Could you check a few things on this model? Use its own coordinates, in mm. A direction names the side the tool comes from. Coordinates: 2 decimals unless noted, no trailing zeros. Order: outer loops, then holes, each group sorted by start corner. A loop starts at its lowest first (then second) coordinate and runs counter-clockwise, first axis right, second up. Notation, with made-up numbers: M 53,-1.75 L 70,-1.75 A27 cw 70,34.25 Z; hole C -15.75,-18 d6. An arc over 180 degrees is marked long. Put each result on its own line as item: value. Start each with the question number.
```python
from build123d import *

# Parameters (mm, degrees)
SKETCH1_R           = 21.5
SKETCH1_R_2         = 1.55
BOSS_EXTRUDE1_DEPTH = 6
SKETCH2_R           = 5.5
SKETCH2_W           = 20
SKETCH2_H           = 10
CUT_EXTRUDE1_DEPTH  = 12
BOSS_EXTRUDE2_DEPTH = 3
SKETCH4_W           = 2
SKETCH4_H           = 4
BOSS_EXTRUDE3_DEPTH = 3
CHAMFER1_SIZE       = 1
CHAMFER2_SIZE       = 3


with BuildPart() as part:
    # Sketch1 → Boss-Extrude1 (new body)
    with BuildSketch(Plane(origin=(0, 0, 0), x_dir=(1, 0, 0), z_dir=(0, 1, 0))):
        with Locations(Location((0, 0, 0), (0, 0, 270))):
            Circle(SKETCH1_R)
        with Locations(Location((0, 17.320762114, 0), (0, 0, 270))):
            Circle(SKETCH1_R_2, mode=Mode.SUBTRACT)
        with Locations(Location((15, -8.66, 0), (0, 0, 270))):
            Circle(SKETCH1_R_2, mode=Mode.SUBTRACT)
        with Locations(Location((-15, -8.66, 0), (0, 0, 270))):
            Circle(SKETCH1_R_2, mode=Mode.SUBTRACT)
    extrude(amount=BOSS_EXTRUDE1_DEPTH)

    # Sketch2 → Cut-Extrude1 (cut)
    with BuildSketch(Plane(origin=(0, 0, 0), x_dir=(-1, 0, 0), z_dir=(0, -1, 0))):
        with Locations(Location((0, 0, 0), (0, 0, 90))):
            Circle(SKETCH2_R)
        with Locations((0, -17)):
            Rectangle(SKETCH2_W, SKETCH2_H)
    extrude(amount=-CUT_EXTRUDE1_DEPTH, mode=Mode.SUBTRACT)

    # Sketch3 → Boss-Extrude2 (add)
    with BuildSketch(Plane(origin=(0, 6, 0), x_dir=(1, 0, 0), z_dir=(0, 1, 0))):
        with BuildLine():
            ThreePointArc((-5.4375, 0.826797285), (-7, 0), (-5.4375, -0.826797285))
            ThreePointArc((-5.4375, -0.826797285), (-5.5, 0), (-5.4375, 0.826797285))
        make_face()
        with BuildLine():
            ThreePointArc((5.4375, -0.826797285), (7, 0), (5.4375, 0.826797285))
            ThreePointArc((5.4375, 0.826797285), (5.5, 0), (5.4375, -0.826797285))
        make_face()
    extrude(amount=BOSS_EXTRUDE2_DEPTH)

    # Sketch4 → Boss-Extrude3 (add)
    with BuildSketch(Plane(origin=(0, 6, 0), x_dir=(1, 0, 0), z_dir=(0, 1, 0))):
        with Locations((8.9375, 0)):
            Rectangle(SKETCH4_W, SKETCH4_H)
    extrude(amount=BOSS_EXTRUDE3_DEPTH)

    # Chamfer1
    chamfer1_edges = [part.edges().sort_by_distance(p)[0] for p in [
        (7.9375, 9, 0),
    ]]
    chamfer(chamfer1_edges, length=CHAMFER1_SIZE)

    # Chamfer2
    chamfer2_edges = [part.edges().sort_by_distance(p)[0] for p in [
        (9.9375, 6, 0),
    ]]
    chamfer(chamfer2_edges, length=CHAMFER2_SIZE - 0.0001)  # a hair under: the kernel refuses the full size


solid = part.part
```
Item 1: For pin 1 Ø1.5 at (y, z) = (3, 2) entering from +X; pin 2 Ø5 at (x, y) = (-5.5, 6.5) entering from -Z; pin 3 Ø5 at (x, y) = (3.5, 3) entering from +Z; pin 4 Ø2.5 at (x, z) = (-15, 8.66) entering from +Y, each with a flat end and sliding along its axis, tell me the tip position at first contact or that it passes through.
Item 2: If we section it at B-B on x = -15.5: Write out the boundary of the cut face in (y, z).
Item 3: For faces 1 (the flat face through (7.938, 7, 0)), 2 (the flat face through (10, 3, 16)), 3 (the flat face through (10, 7, 2)), 4 (the flat face through (10, 7, -2)), 5 (the cylindrical face through (7, 7, 0)), which set-ups out of +Z, -Z, +X, -X, +Y, -Y let a thin tool reach every point of the face, with its end or its side?
Item 4: If we section it at A-A on y = 1.5: Write out the boundary of the cut face in (x, z), then the cut area to 3 significant figures.
Item 5: If we mould it in two halves opening along X, with no side actions, what happens to faces 6 (the cylindrical face through (0.07, 2.96, -18.87)), 7 (the flat face through (11.42, 7.52, 0.03)), 8 (the flat face through (0, 0, -6))? For each: released by +X, released by -X, zero draft, split by the parting line, or undercut.
Item 6: If we section it at D-D on y = 8.5: Write out the boundary of the cut face in (x, z), then the cut area to 3 significant figures.
Item 7: If we section it at C-C on z = 9: Write out the boundary of the cut face in (x, y), then the cut area to 3 significant figures.
Item 8: I need wall thicknesses on probe 1 along X at (y, z) = (3.8, 8.66); probe 2 along X at (y, z) = (1.65, 0); probe 3 along Y at (x, z) = (7, 8). Which ranges of each line are inside material? Lowest first, please.
Geometry check:
1. pin 1: stops at x = 21.46
1. pin 2: stops at z = -21.28
1. pin 3: stops at z = 12
1. pin 4: passes through
2. outline: M 0,-14.9 L 6,-14.9 L 6,7.19 L 0,7.19 Z; M 0,10.13 L 6,10.13 L 6,14.9 L 0,14.9 Z
3. face 1: +Z, -Z, +Y
3. face 2: +Z, +Y, -Y
3. face 3: +Z, +X, -X, +Y
3. face 4: -Z, +X, -X, +Y
3. face 5: +Y
4. outline: M -10,12 L -10,19.03 A21.5 ccw long 10,19.03 L 10,12 Z; hole C -15,8.66 d3.1; hole C 0,0 d11; hole C 0,-17.32 d3.1; hole C 15,8.66 d3.1
4. area: 1,160 mm²
5. face 6: undercut
5. face 7: released by +X
5. face 8: zero draft
6. outline: M -5.44,-0.83 A5.5 cw -5.44,0.83 A1 ccw long Z; M 5.44,-0.83 A1 ccw long 5.44,0.83 A5.5 cw Z; M 8.44,-2 L 10.44,-2 L 10.44,2 L 8.44,2 Z
6. area: 13.1 mm²
7. outline: M -19.53,0 L -16.51,0 L -16.51,6 L -19.53,6 Z; M -13.49,0 L 13.49,0 L 13.49,6 L -13.49,6 Z; M 16.51,0 L 19.53,0 L 19.53,6 L 16.51,6 Z
7. area: 198 mm²
8. probe 1: x = -19.68 to -16.55, -13.45 to 13.45, 16.55 to 19.68
8. probe 2: x = -21.5 to -5.5, 5.5 to 21.5
8. probe 3: y = 0 to 6
